Part model, mm, in its own coordinate system. A direction names the side the tool comes from. Coordinates: 2 decimals unless noted, no trailing zeros. Write each loop counter-clockwise with the first axis right and the second up, starting at its lowest first coordinate (ties: lowest second). Pieces come first, ordered by that corner, then holes. Notation, with made-up numbers: (20.25, -35) -> (43.25, -35) arc R36 cw to (43.25, 0) -> close; hole circle Ø7 at (-39, 11.5). An arc over 180 degrees is marked (long way). Write item = value, one per line. Start each with the question number.
Q1. Tool access for faces 5 (the flat face through (-39.656, -14.79, -9.88)), 6 (the flat face through (-27.865, -14.79, -2.244)): list every direction of +Z, -Z, +X, -X, +Y, -Y with a clear straight run to the whole face (end or side of a thin tool).
Q2. Band-saw the part on A-A, the plane y = -18. List the corners of the cut face in (x, z), plus the area to 3 significant figures.
Q3. Probe line 1 (Z direction, x = 25, y = -20); line 2 (X direction, y = -7.75, z = 0); line 3 (X direction, y = -11.25, z = 21.5). List the from-to ranges inside material, lowest first.
Q4. Band-saw the part on B-B, the plane z = 6. List the corners of the cut face in (x, y).
Q5. Pin check, flat tips, straight feed: P1, Ø8, axis at y = -8.5, z = -22, coming from the -X side; P2, Ø8, axis at y = -23, z = -43, coming from the -X side; P3, Ø12, axis at x = -34.5, y = -11, coming from the -Z side. Stop position of each tip, or through.
Q6. Band-saw the part on D-D, the plane x = 18. List the corners of the cut face in (y, z), plus the area to 3 significant figures.
Q7. Pull direction X, two halves, no side cores. Call faces 1 (the flat face through (19, -30, 5)), 2 (the flat face through (78.655, -14.79, 19.477)), 3 (the flat face through (40.504, -14.79, -46.237)), 4 (the flat face through (-54.954, -14.79, 63.859)): released by +X, released by -X, zero draft, split by the parting line, or undercut.
Q8. Band-saw the part on C-C, the plane x = 46.5. List the corners of the cut face in (y, z), plus the area to 3 significant figures.
from build123d import *

# Parameters (mm, degrees)
F1_DEPTH = 30


with BuildPart() as f1:
    # F0 (on Front) → F1 (new body)
    with BuildSketch(Plane.XZ):
        Polygon((52.768022, 57.033721), (-44.317942, 78.629129), (-65.8926, 48.668932), (-12.675109, -70.090957), (83.332121, -53.882539), (103.828043, -17.042199), align=None)
        Polygon((4.225037, -53.882539), (52.768022, 33.813149), (87.822262, -17.042199), (75.780988, -38.802642), align=None, mode=Mode.SUBTRACT)
        Polygon((-47.554146, 43.428849), (-38.205128, 65.291479), (38.025331, 43.428849), (-8.719755, -46.655327), align=None, mode=Mode.SUBTRACT)
    extrude(amount=F1_DEPTH)


solid = f1.part
Ans:
q1.face_5 = -Z, -X, +Y, -Y
q1.face_6 = +Y, -Y
q2.outline = (-65.89, 48.67) -> (-12.68, -70.09) -> (83.33, -53.88) -> (103.83, -17.04) -> (52.77, 57.03) -> (-44.32, 78.63) -> close; hole (-47.55, 43.43) -> (-8.72, -46.66) -> (38.03, 43.43) -> (-38.21, 65.29) -> close; hole (4.23, -53.88) -> (75.78, -38.8) -> (87.82, -17.04) -> (52.77, 33.81) -> close
q2.area = 7,980 mm2
q3.line_1 = -63.73 to -49.5, -16.35 to 18.33, 47.16 to 63.21
q3.line_2 = -44.08 to -28.83, 15.49 to 34.05, 76.08 to 92.08
q3.line_3 = -53.72 to -38.1, 26.65 to 45.95, 61.26 to 77.26
q4.outline = (-46.77, -30) -> (-31.42, -30) -> (-31.42, 0) -> (-46.77, 0) -> close; (18.6, -30) -> (37.37, -30) -> (37.37, 0) -> (18.6, 0) -> close; (71.94, -30) -> (87.95, -30) -> (87.95, 0) -> (71.94, 0) -> close
q5.P1 = -36.02
q5.P2 = -26.61
q5.P3 = -34.78
q6.outline = (-30, -64.91) -> (0, -64.91) -> (0, -50.98) -> (-30, -50.98) -> close; (-30, -29) -> (0, -29) -> (0, 4.84) -> (-30, 4.84) -> close; (-30, 49.17) -> (0, 49.17) -> (0, 64.77) -> (-30, 64.77) -> close
q6.area = 1,900 mm2
q7.face_1 = zero draft
q7.face_2 = released by +X
q7.face_3 = undercut
q7.face_4 = released by -X
q8.outline = (-30, -60.1) -> (0, -60.1) -> (0, -44.97) -> (-30, -44.97) -> close; (-30, 22.49) -> (0, 22.49) -> (0, 58.43) -> (-30, 58.43) -> close
q8.area = 1,530 mm2
